from build123d import *

# Parameters (mm, degrees)
SKETCH_1_W          = 30
SKETCH_1_H          = 24
EXTRUDE_1_DEPTH     = 2
EXTRUDE_2_DEPTH     = 3
SKETCH_3_W          = 3
SKETCH_3_H          = 3
EXTRUDE_3_DEPTH     = 2
SKETCH_4_W          = 24
SKETCH_4_H          = 2
EXTRUDE_4_DEPTH     = 8.5
SKETCH_5_W          = 5.5
SKETCH_5_H          = 10.5
SKETCH_5_W_2        = 3.5
SKETCH_5_H_2        = 8.5
EXTRUDE_5_DEPTH     = 8
SKETCH_6_W          = 1
SKETCH_6_H          = 6.5
CUT_EXTRUDE_1_DEPTH = 8
SKETCH_7_W          = 8.5
SKETCH_7_H          = 5.5
CUT_EXTRUDE_2_DEPTH = 9
SKETCH_8_W          = 8
SKETCH_8_H          = 7
SKETCH_8_R          = 2.4
EXTRUDE_6_DEPTH     = 2


with BuildPart() as part:
    # 草图1 → 凸台-拉伸1 (new body)
    with BuildSketch(Plane(origin=(0, 0, 0), x_dir=(1, 0, 0), z_dir=(0, 1, 0))):
        Rectangle(SKETCH_1_W, SKETCH_1_H)
    extrude(amount=EXTRUDE_1_DEPTH)

    # 草图2 → 凸台-拉伸2 (add)
    with BuildSketch(Plane(origin=(0, 2, 0), x_dir=(1, 0, 0), z_dir=(0, 1, 0))):
        Polygon((-15, 12), (-15, 6), (-12.75, 6), (-12.75, 9), (-9.75, 9), (-9.75, 12), align=None)
        Polygon((9.75, 12), (15, 12), (15, 6), (12.75, 6), (12.75, 9), (9.75, 9), align=None)
        Polygon((15, -12), (15, -6), (12.75, -6), (12.75, -9), (9.75, -9), (9.75, -12), align=None)
        Polygon((-9.75, -12), (-15, -12), (-15, -6), (-12.75, -6), (-12.75, -9), (-9.75, -9), align=None)
    extrude(amount=EXTRUDE_2_DEPTH)

    # 草图3 → 凸台-拉伸3 (add)
    with BuildSketch(Plane(origin=(0, 2, 0), x_dir=(1, 0, 0), z_dir=(0, 1, 0))):
        with Locations((-11.25, 7.5)):
            Rectangle(SKETCH_3_W, SKETCH_3_H)
        with Locations((11.25, 7.5)):
            Rectangle(SKETCH_3_W, SKETCH_3_H)
        with Locations((11.25, -7.5)):
            Rectangle(SKETCH_3_W, SKETCH_3_H)
        with Locations((-11.25, -7.5)):
            Rectangle(SKETCH_3_W, SKETCH_3_H)
    extrude(amount=EXTRUDE_3_DEPTH)

    # 草图4 → 凸台-拉伸4 (add)
    with BuildSketch(Plane(origin=(15, 0, 0), x_dir=(0, 0, -1), z_dir=(1, 0, 0))):
        with Locations((0, 1)):
            Rectangle(SKETCH_4_W, SKETCH_4_H)
    extrude(amount=EXTRUDE_4_DEPTH)

    # 草图5 → 凸台-拉伸5 (add)
    with BuildSketch(Plane(origin=(0, 2, 0), x_dir=(1, 0, 0), z_dir=(0, 1, 0))):
        with Locations((20.75, 0)):
            Rectangle(SKETCH_5_W, SKETCH_5_H)
        with Locations((20.75, 0)):
            Rectangle(SKETCH_5_W_2, SKETCH_5_H_2, mode=Mode.SUBTRACT)
    extrude(amount=EXTRUDE_5_DEPTH)

    # 草图6 → 切除-拉伸1 (cut)
    with BuildSketch(Plane(origin=(0, 10, 0), x_dir=(1, 0, 0), z_dir=(0, 1, 0))):
        with Locations((23, 0)):
            Rectangle(SKETCH_6_W, SKETCH_6_H)
    extrude(amount=-CUT_EXTRUDE_1_DEPTH, mode=Mode.SUBTRACT)

    # 草图7 → 切除-拉伸2 (cut)
    with BuildSketch(Plane(origin=(0, 2, 0), x_dir=(1, 0, 0), z_dir=(0, 1, 0))):
        with Locations((19.25, 9.25)):
            Rectangle(SKETCH_7_W, SKETCH_7_H)
        with Locations((19.25, -9.25)):
            Rectangle(SKETCH_7_W, SKETCH_7_H)
    extrude(amount=-CUT_EXTRUDE_2_DEPTH, mode=Mode.SUBTRACT)

    # 草图8 → 凸台-拉伸6 (add)
    # profile 1 of 2: a face of its own
    with BuildSketch(Plane(origin=(0, 2, 0), x_dir=(1, 0, 0), z_dir=(0, 1, 0))):
        with Locations((4, -15.5)):
            Rectangle(SKETCH_8_W, SKETCH_8_H)
        with Locations(Location((4, -15, 0), (0, 0, 270))):
            Circle(SKETCH_8_R, mode=Mode.SUBTRACT)
    # profile 2 of 2: a face of its own
    with BuildSketch(Plane(origin=(0, 2, 0), x_dir=(1, 0, 0), z_dir=(0, 1, 0))):
        with Locations((4, 15.5)):
            Rectangle(SKETCH_8_W, SKETCH_8_H)
        with Locations(Location((4, 15, 0), (0, 0, 270))):
            Circle(SKETCH_8_R, mode=Mode.SUBTRACT)
    extrude(amount=-EXTRUDE_6_DEPTH)


solid = part.part
Design review of the part built by this model. Coordinates are the model's own, in mm. A direction names the side the tool comes from. Round coordinates to 2 decimals unless told otherwise and drop trailing zeros. Write each loop counter-clockwise with the first axis right and the second up, starting at its lowest first coordinate (ties: lowest second). Pieces come first, ordered by that corner, then holes. Notation, with made-up numbers: (77, -19) -> (87, -19) arc R26 cw to (87, 6) -> close; hole circle Ø5 at (73, 51.25). An arc over 180 degrees is marked (long way). One line per question, with ' | ' between items.
(1) Insertion check: P1, Ø0.6, axis at y = 1, z = 15.5, coming from the -X side; P2, Ø0.9, axis at x = 10.5, z = 7.5, coming from the +Y side; P3, Ø10, axis at x = 10.5, z = -6, coming from the +Y side. Each pin has a flat end and moves straight along its axis. Give the tip position at first contact, or say it passes through.
Result sheet:
P1: x = 0 | P2: y = 4 | P3: y = 5
(2) Take a section at B-B, the plane y = 3.5. State the section outline as (x, z) points.
Result sheet:
outline: (-15, -12) -> (-9.75, -12) -> (-9.75, -6) -> (-15, -6) -> close; (-15, 6) -> (-9.75, 6) -> (-9.75, 12) -> (-15, 12) -> close; (9.75, -12) -> (15, -12) -> (15, -6) -> (9.75, -6) -> close; (9.75, 6) -> (15, 6) -> (15, 12) -> (9.75, 12) -> close; (18, -5.25) -> (23.5, -5.25) -> (23.5, -3.25) -> (22.5, -3.25) -> (22.5, -4.25) -> (19, -4.25) -> (19, 4.25) -> (22.5, 4.25) -> (22.5, 3.25) -> (23.5, 3.25) -> (23.5, 5.25) -> (18, 5.25) -> close
(3) Take a section at C-C, the plane x = 4. State the section outline as (y, z) points, and give its area (3 significant figures).
Result sheet:
outline: (0, -19) -> (2, -19) -> (2, -17.4) -> (0, -17.4) -> close; (0, -12.6) -> (2, -12.6) -> (2, 12.6) -> (0, 12.6) -> close; (0, 17.4) -> (2, 17.4) -> (2, 19) -> (0, 19) -> close | area: 56.8 mm2
(4) Wall thickness on line 1 (X direction, y = 0.9, z = -15); line 2 (Z direction, x = 20.5, y = 4); line 3 (X direction, y = 5.5, z = 4): over which ranges is each line inside the solid? List them lowest first. Write a range as [from, to].
Result sheet:
line 1: [0, 1.6], [6.4, 8] | line 2: [-5.25, -4.25], [4.25, 5.25] | line 3: [18, 19], [22.5, 23.5]
(5) Machinability: for faces 4 (the flat face through (12, 3, 6)), 5 (the flat face through (23, 6, -3.25)), 6 (the flat face through (9.75, 3, 9)), which of the approach directions +Z, -Z, +X, -X, +Y, -Y give a long, thin tool a straight path to every point of the face, cutting with its end or side? Answer none if there is none.
Result sheet:
face 4: +X, -X, +Y | face 5: +X, +Y | face 6: +Z, -Z, +Y
(6) Draft analysis for pull direction Z (two halves, no side actions). For faces 1 (the flat face through (-12, 3, 6)), 2 (the flat face through (15, 3, -9)), 3 (the flat face through (21, 6, -5.25)), state which applies: released by +Z, released by -Z, zero draft, split by the parting line, or undercut.
Result sheet:
face 1: undercut | face 2: zero draft | face 3: released by -Z
(7) Take a section at A-A, the plane z = -15. State the section outline as (x, y) points.
Result sheet:
outline: (0, 0) -> (1.6, 0) -> (1.6, 2) -> (0, 2) -> close; (6.4, 0) -> (8, 0) -> (8, 2) -> (6.4, 2) -> close
(8) Take a section at D-D, the plane y = 1.25. State the section outline as (x, z) points.
Result sheet:
outline: (-15, -12) -> (0, -12) -> (0, -19) -> (8, -19) -> (8, -12) -> (15, -12) -> (15, -6.5) -> (23.5, -6.5) -> (23.5, 6.5) -> (15, 6.5) -> (15, 12) -> (8, 12) -> (8, 19) -> (0, 19) -> (0, 12) -> (-15, 12) -> close; hole circle Ø4.8 at (4, -15); hole circle Ø4.8 at (4, 15)
